```python
from build123d import *

# Parameters (mm, degrees)
BOSS_EXTRUDE1_DEPTH     = 9.525
SKETCH2_W               = 94.331668948
SKETCH2_H               = 25.4
CUT_EXTRUDE1_DEPTH      = 254.880909582
FILLET1_R               = 6.35
FILLET2_R               = 6.35
F_1_4_CLEARANCE_HOLE1_D = 6.7564


with BuildPart() as part:
    # Sketch1 → Boss-Extrude1 (new body)
    with BuildSketch(Plane(origin=(0, 0, 0), x_dir=(1, 0, 0), z_dir=(0, 1, 0))):
        with BuildLine():
            Line((28.575, 81.75625), (28.575, 160.782))
            Line((28.575, 160.782), (0, 160.782))
            Line((0, 160.782), (0, 0))
            Line((0, 0), (82.55, 0))
            Line((82.55, 0), (118.11, 120.65))
            Line((118.11, 120.65), (118.11, 139.7))
            ThreePointArc((118.11, 139.7), (139.7, 161.29), (161.29, 139.7))
            Line((161.29, 139.7), (161.29, 120.65))
            Line((161.29, 120.65), (180.975, 120.65))
            Line((180.975, 120.65), (180.975, 139.7))
            Line((180.975, 139.7), (180.975, 177.8))
            Line((180.975, 177.8), (121.7041, 177.8))
            Line((121.7041, 177.8), (80.9625, 177.8))
            Line((80.9625, 177.8), (80.9625, 81.75625))
            ThreePointArc((80.9625, 81.75625), (54.76875, 55.5625), (28.575, 81.75625))
        make_face()
    extrude(amount=BOSS_EXTRUDE1_DEPTH)

    # Sketch2 → Cut-Extrude1 (cut, through all)
    with BuildSketch(Plane(origin=(0, 9.525, 0), x_dir=(1, 0, 0), z_dir=(0, 1, 0))):
        with Locations((47.165834474, 12.7)):
            Rectangle(SKETCH2_W, SKETCH2_H)
    extrude(amount=-CUT_EXTRUDE1_DEPTH, mode=Mode.SUBTRACT)

    # Fillet1
    fillet1_edges = [part.edges().sort_by_distance(p)[0] for p in [
        (0, 4.7625, -25.4),
    ]]
    fillet(fillet1_edges, radius=FILLET1_R)

    # Fillet2
    fillet2_edges = [part.edges().sort_by_distance(p)[0] for p in [
        (0, 4.7625, -160.782),
        (180.975, 4.7625, -177.8),
        (180.975, 4.7625, -120.65),
        (90.036315789, 4.7625, -25.4),
    ]]
    fillet(fillet2_edges, radius=FILLET2_R)

    # 1/4 Clearance Hole1 (through all)
    with Locations(Plane(origin=(0, 9.525, 0), x_dir=(1, 0, 0), z_dir=(0, 1, 0))):
        with Locations((14.2875, 146.05), (14.2875, 44.45), (99.2378, 146.05), (170.92295, 146.05)):
            Hole(F_1_4_CLEARANCE_HOLE1_D / 2)


solid = part.part
```
Work out the finished part from the listing and answer in its coordinate system (mm). A direction names the side the tool comes from. Give positions to 0.01 mm unless a question says otherwise; leave off trailing zeros. Write each loop counter-clockwise with the first axis right and the second up, starting at its lowest first coordinate (ties: lowest second). Pieces come first, ordered by that corner, then holes. Notation, with made-up numbers: (76, -20) - (103, -20) arc R24 ccw to (103, 2) - close; hole circle Ø11 at (-33, 15.25). An arc over 180 degrees is marked (long way). Use one line per item in the form item = value.
1. A cutting plane is placed at B-B (y = 4). State how many separate pieces and enclosed holes the cut face has, and give its area (3 significant figures).
Filled in:
separate_pieces = 1
enclosed_holes = 4
area = 11,900 mm^2
2. A cutting plane is placed at A-A (z = -44.45). Write down the section's boundary in (x, y) (3 decimals), and give its area (3 significant figures).
Filled in:
outline = (0, 0) - (10.909, 0) - (10.909, 9.525) - (0, 9.525) - close; (17.666, 0) - (95.651, 0) - (95.651, 9.525) - (17.666, 9.525) - close
area = 847 mm^2
3. A cutting plane is placed at D-D (x = 139.7). Write down the section's boundary in (y, z) (3 decimals).
Filled in:
outline = (0, -177.8) - (9.525, -177.8) - (9.525, -161.29) - (0, -161.29) - close
4. A cutting plane is placed at C-C (z = -146.05). Write down the section's boundary in (x, y) (1 decimal), and give its area (3 significant figures).
Filled in:
outline = (0, 0) - (10.9, 0) - (10.9, 9.5) - (0, 9.5) - close; (17.7, 0) - (28.6, 0) - (28.6, 9.5) - (17.7, 9.5) - close; (81, 0) - (95.9, 0) - (95.9, 9.5) - (81, 9.5) - close; (102.6, 0) - (119.1, 0) - (119.1, 9.5) - (102.6, 9.5) - close; (160.3, 0) - (167.5, 0) - (167.5, 9.5) - (160.3, 9.5) - close; (174.3, 0) - (181, 0) - (181, 9.5) - (174.3, 9.5) - close
area = 639 mm^2
5. Each of these flat-tipped pins is pushed along its axis until it touches: pin 1 Ø3 at (x, y) = (165.5, 5.5) entering from +Z; pin 2 Ø5 at (x, y) = (17.5, 2.5) entering from -Z; pin 3 Ø2 at (y, z) = (3.5, -90.5) entering from +X. Where does it stop, or does it pass through?
Filled in:
pin_1 = -120.65
pin_2 = -160.78
pin_3 = 109.52
6. Determine the mould class of faces 6 (the face through (55.34, 4.7, -55.57)), 7 (the face through (89, 0, -103)), 8 (the face through (173.6, 4.7, -143.99)) for opening direction Z: released by +Z, released by -Z, zero draft, split by the parting line, or undercut.
Filled in:
face_6 = released by -Z
face_7 = zero draft
face_8 = undercut
7. For faces 1 (the face through (128, 5, -177.8)), 2 (the face through (168, 5, -120.65)), 3 (the face through (15.02, 4.696, -142.752)), 4 (the face through (80.962, 5, -130)), 5 (the face through (161.29, 5, -130)), determine the directions among +Z, -Z, +X, -X, +Y, -Y from which every point of the face is accessible in a straight line to the end or side of a thin tool.
Filled in:
face_1 = -Z, +X, -X, +Y, -Y
face_2 = +Z, +X, +Y, -Y
face_3 = +Y, -Y
face_4 = -Z, +Y, -Y
face_5 = +Z, +Y, -Y
8. Consider L1, parallel to X at y = 6, z = -146.05 (1 decimal); L2, parallel to X at y = 8.5, z = -151 (1 decimal); L3, parallel to Z at x = 12.5, y = 1.5. Determine where each line is inside the solid, lowest interval first.
Filled in:
L1 = 0 to 10.9, 17.7 to 28.6, 81 to 95.9, 102.6 to 119.1, 160.3 to 167.5, 174.3 to 181
L2 = 0 to 28.6, 81 to 121.3, 158.1 to 181
L3 = -160.78 to -148.92, -143.18 to -47.32, -41.58 to -25.4
